Geometry: final body of the model. Coordinates: model frame, mm. Round coordinates to 2 decimals unless told otherwise and drop trailing zeros. Loops run counter-clockwise (first coordinate to the right, second up) from the corner with the lowest first, then second, coordinate; pieces in that order, holes last. Notation, with made-up numbers: M -16,64.25 L -11,64.25 A24 cw -11,90.25 Z; hole C 47,74.25 d2. An arc over 180 degrees is marked long. Write each question's results on one line, items separated by ' | '.
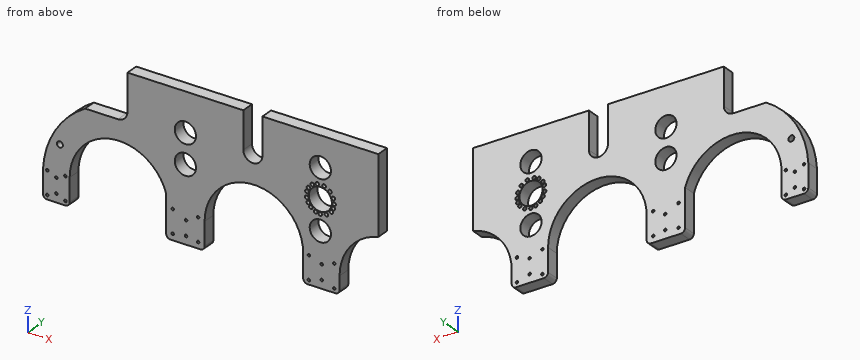
```python
from build123d import *

# Parameters (mm, degrees)
SKETCH3_R           = 7
SKETCH3_R_2         = 3
SKETCH3_R_3         = 25.1
SKETCH3_R_4         = 27.215273825
SKETCH3_R_5         = 4.25
BOSS_EXTRUDE2_DEPTH = 30


with BuildPart() as part:
    # Sketch3 → Boss-Extrude2 (new body)
    with BuildSketch(Plane(origin=(0, 0, 0), x_dir=(1, 0, 0), z_dir=(0, 1, 0))):
        with BuildLine():
            Line((0, 0), (273.87, 0))
            Line((273.87, 0), (273.87, 87.5))
            ThreePointArc((273.87, 87.5), (296.37, 110), (318.87, 87.5))
            Line((318.87, 87.5), (318.87, 0))
            Line((318.87, 0), (592.74, 0))
            Line((592.74, 0), (592.74, 183.19))
            ThreePointArc((592.74, 183.19), (526.952473324, 223.969990415), (501.24, 296.97598332))
            Line((501.24, 296.97598332), (501.24, 328.489999343))
            ThreePointArc((501.24, 328.489999343), (498.311067812, 335.561067155), (491.24, 338.489999343))
            Line((491.24, 338.489999343), (425.37, 338.489999343))
            ThreePointArc((425.37, 338.489999343), (418.298932188, 335.561067155), (415.37, 328.489999343))
            Line((415.37, 328.489999343), (415.37, 273.489999343))
            ThreePointArc((415.37, 273.489999343), (298.87, 156.989999343), (182.37, 273.489999343))
            Line((182.37, 273.489999343), (182.37, 328.489999343))
            ThreePointArc((182.37, 328.489999343), (179.441067812, 335.561067155), (172.37, 338.489999343))
            Line((172.37, 338.489999343), (101.5, 338.489999343))
            ThreePointArc((101.5, 338.489999343), (94.428932188, 335.561067155), (91.5, 328.489999343))
            Line((91.5, 328.489999343), (91.5, 239.726113311))
            ThreePointArc((91.5, 239.726113311), (-37.066048166, 158.246778284), (-136.5, 273.489999343))
            Line((-136.5, 273.489999343), (-136.5, 328.489999343))
            ThreePointArc((-136.5, 328.489999343), (-139.428932188, 335.561067155), (-146.5, 338.489999343))
            Line((-146.5, 338.489999343), (-189.5, 338.489999343))
            ThreePointArc((-189.5, 338.489999343), (-196.571067812, 335.561067155), (-199.5, 328.489999343))
            Line((-199.5, 328.489999343), (-199.5, 273.489999343))
            ThreePointArc((-199.5, 273.489999343), (-170.358013315, 179.208137798), (-100.012022841, 109.999999343))
            Line((-100.012022841, 109.999999343), (-22.509563758, 109.999999343))
            ThreePointArc((-22.509563758, 109.999999343), (-6.60053067, 103.410771361), (-0.009563892, 87.50245856))
            Line((-0.009563892, 87.50245856), (0, 0))
        make_face()
        with Locations(Location((-159.5, 207.499999343, 0), (0, 0, 270))):
            Circle(SKETCH3_R, mode=Mode.SUBTRACT)
        with Locations(Location((-189.5, 328.489999343, 0), (0, 0, 270))):
            Circle(SKETCH3_R_2, mode=Mode.SUBTRACT)
        with Locations(Location((-146.5, 328.489999343, 0), (0, 0, 270))):
            Circle(SKETCH3_R_2, mode=Mode.SUBTRACT)
        with Locations(Location((-167.860538183, 318.489999343, 0), (0, 0, 270))):
            Circle(SKETCH3_R_2, mode=Mode.SUBTRACT)
        with Locations(Location((-146.5, 273.489999343, 0), (0, 0, 270))):
            Circle(SKETCH3_R_2, mode=Mode.SUBTRACT)
        with Locations(Location((-167.860538183, 283.489999343, 0), (0, 0, 270))):
            Circle(SKETCH3_R_2, mode=Mode.SUBTRACT)
        with Locations(Location((-189.5, 273.489999343, 0), (0, 0, 270))):
            Circle(SKETCH3_R_2, mode=Mode.SUBTRACT)
        with Locations(Location((166.986079988, 269.062698156, 0), (0, 0, 270))):
            Circle(SKETCH3_R_2, mode=Mode.SUBTRACT)
        with Locations(Location((166.986079988, 323.925123651, 0), (0, 0, 270))):
            Circle(SKETCH3_R_2, mode=Mode.SUBTRACT)
        with Locations(Location((138.449645935, 319.171398702, 0), (0, 0, 270))):
            Circle(SKETCH3_R_2, mode=Mode.SUBTRACT)
        with Locations(Location((106.986375646, 269.062698156, 0), (0, 0, 270))):
            Circle(SKETCH3_R_2, mode=Mode.SUBTRACT)
        with Locations(Location((106.986375646, 323.736765186, 0), (0, 0, 270))):
            Circle(SKETCH3_R_2, mode=Mode.SUBTRACT)
        with Locations(Location((488.822646039, 273.49, 0), (0, 0, 270))):
            Circle(SKETCH3_R_2, mode=Mode.SUBTRACT)
        with Locations(Location((488.822646039, 328.49, 0), (0, 0, 270))):
            Circle(SKETCH3_R_2, mode=Mode.SUBTRACT)
        with Locations(Location((459.034690833, 319.171398702, 0), (0, 0, 270))):
            Circle(SKETCH3_R_2, mode=Mode.SUBTRACT)
        with Locations(Location((428.822646039, 273.49, 0), (0, 0, 270))):
            Circle(SKETCH3_R_2, mode=Mode.SUBTRACT)
        with Locations(Location((428.822646039, 328.49, 0), (0, 0, 270))):
            Circle(SKETCH3_R_2, mode=Mode.SUBTRACT)
        with Locations(Location((138.449645935, 284.171398702, 0), (0, 0, 270))):
            Circle(SKETCH3_R_2, mode=Mode.SUBTRACT)
        with Locations(Location((459.034690833, 284.171398702, 0), (0, 0, 270))):
            Circle(SKETCH3_R_2, mode=Mode.SUBTRACT)
        with Locations(Location((136.93, 161.5, 0), (0, 0, 270))):
            Circle(SKETCH3_R_3, mode=Mode.SUBTRACT)
        with Locations(Location((136.93, 91.5, 0), (0, 0, 270))):
            Circle(SKETCH3_R_3, mode=Mode.SUBTRACT)
        with Locations(Location((455.81, 211.5, 0), (0, 0, 270))):
            Circle(SKETCH3_R_3, mode=Mode.SUBTRACT)
        with Locations(Location((455.81, 71.5, 0), (0, 0, 270))):
            Circle(SKETCH3_R_3, mode=Mode.SUBTRACT)
        with Locations(Location((455.81, 141.5, 0), (0, 0, 270))):
            Circle(SKETCH3_R_4, mode=Mode.SUBTRACT)
        with Locations(Location((455.81, 174.25, 0), (0, 0, 270))):
            Circle(SKETCH3_R_5, mode=Mode.SUBTRACT)
        with Locations(Location((470.12937162, 170.953660153, 0), (0, 0, 270))):
            Circle(SKETCH3_R_5, mode=Mode.SUBTRACT)
        with Locations(Location((481.743809978, 161.5, 0), (0, 0, 270))):
            Circle(SKETCH3_R_5, mode=Mode.SUBTRACT)
        with Locations(Location((486.641730392, 152.543862595, 0), (0, 0, 270))):
            Circle(SKETCH3_R_5, mode=Mode.SUBTRACT)
        with Locations(Location((488.54728895, 142.41236627, 0), (0, 0, 270))):
            Circle(SKETCH3_R_5, mode=Mode.SUBTRACT)
        with Locations(Location((486.641730392, 130.456137405, 0), (0, 0, 270))):
            Circle(SKETCH3_R_5, mode=Mode.SUBTRACT)
        with Locations(Location((478.633688814, 117.855315192, 0), (0, 0, 270))):
            Circle(SKETCH3_R_5, mode=Mode.SUBTRACT)
        with Locations(Location((464.525450227, 109.930973608, 0), (0, 0, 270))):
            Circle(SKETCH3_R_5, mode=Mode.SUBTRACT)
        with Locations(Location((448.462502984, 109.584850187, 0), (0, 0, 270))):
            Circle(SKETCH3_R_5, mode=Mode.SUBTRACT)
        with Locations(Location((437.02438353, 114.673462507, 0), (0, 0, 270))):
            Circle(SKETCH3_R_5, mode=Mode.SUBTRACT)
        with Locations(Location((427.857640986, 124.434592722, 0), (0, 0, 270))):
            Circle(SKETCH3_R_5, mode=Mode.SUBTRACT)
        with Locations(Location((424.022707805, 133.61770624, 0), (0, 0, 270))):
            Circle(SKETCH3_R_5, mode=Mode.SUBTRACT)
        with Locations(Location((423.572722, 147.036738763, 0), (0, 0, 270))):
            Circle(SKETCH3_R_5, mode=Mode.SUBTRACT)
        with Locations(Location((427.166538269, 157.378117019, 0), (0, 0, 270))):
            Circle(SKETCH3_R_5, mode=Mode.SUBTRACT)
        with Locations(Location((433.541295108, 165.513897694, 0), (0, 0, 270))):
            Circle(SKETCH3_R_5, mode=Mode.SUBTRACT)
        with Locations(Location((444.546820962, 172.252289312, 0), (0, 0, 270))):
            Circle(SKETCH3_R_5, mode=Mode.SUBTRACT)
    extrude(amount=BOSS_EXTRUDE2_DEPTH)


solid = part.part
```
1. Pin query (flat end, axial travel): P1, Ø5, axis at x = 459.03, z = -319.17, coming from the -Y side; P2, Ø10, axis at x = -8.5, y = 18, coming from the -Z side; P3, Ø1.5, axis at y = 8, z = -233.5, coming from the -X side; P4, Ø8, axis at y = 5.5, z = -165.5, coming from the -X side. Return the tip coordinate at first contact, or that it passes through.
Answer key:
P1: passes through | P2: stops at z = -158.16 | P3: stops at x = -193.52 | P4: stops at x = -164.06
2. Ray query, probe 1 along X at (y, z) = (4.25, -310.5); probe 2 along X at (y, z) = (20.75, -71.5); probe 3 along X at (y, z) = (18.25, -154). Return the intervals inside material, ascending.
Answer key:
probe 1: x = -199.5 to -136.5, 91.5 to 182.37, 415.37 to 501.24 | probe 2: x = -0.01 to 121.76, 152.1 to 273.87, 318.87 to 430.71, 480.91 to 592.74 | probe 3: x = -152.22 to 112.98, 160.88 to 424.59, 429.75 to 431.64, 479.98 to 482.65, 490.63 to 592.74
3. Section B-B (x = 227.5). Output: boundary loops of the cut face in (y, z).
Answer key:
outline: M 0,-181.41 L 30,-181.41 L 30,0 L 0,0 Z
4. Section A-A (y = 18). Count the separate pieces of the cut face and the enclosed holes in it, then the cut area to 3 significant figures.
Answer key:
separate pieces: 1 | enclosed holes: 40 | area: 141,000 mm²
5. Section C-C (x = -63). Output: boundary loops of the cut face in (y, z).
Answer key:
outline: M 0,-165.22 L 30,-165.22 L 30,-110 L 0,-110 Z
